from build123d import *

# Parameters (mm, degrees)
SKETCH1_R           = 20
SKETCH1_R_2         = 10
BOSS_EXTRUDE1_DEPTH = 10
SKETCH5_R           = 16.925
BOSS_EXTRUDE2_DEPTH = 20
BOSS_EXTRUDE3_DEPTH = 40
CIRPATTERN1_COUNT   = 4


with BuildPart() as part:
    # Sketch1 → Boss-Extrude1 (new, symmetric)
    with BuildSketch(Plane.XY):
        Circle(SKETCH1_R)
        Circle(SKETCH1_R_2, mode=Mode.SUBTRACT)
    extrude(amount=BOSS_EXTRUDE1_DEPTH, both=True)

    # Sketch5 → Boss-Extrude2 (add, symmetric)
    with BuildSketch(Plane.XY.offset(10)):
        Circle(SKETCH5_R)
    extrude(amount=BOSS_EXTRUDE2_DEPTH, both=True)

    # Sketch6 → Boss-Extrude3 (add)
    with BuildSketch(Plane(origin=(0, 0, 0), x_dir=(0, 0, -1), z_dir=(1, 0, 0))):
        Polygon((10, 0), (-10, 20), (-10, 17), (10, -3), align=None)
    boss_extrude3 = extrude(amount=BOSS_EXTRUDE3_DEPTH)

    # CirPattern1: Boss-Extrude3 ×4 about axis
    cirpattern1_axis = Axis((1.370302178, -0.068730139, 0), (0, 0, 1))
    for i in range(1, CIRPATTERN1_COUNT):
        add(boss_extrude3.rotate(cirpattern1_axis, i * 360 / CIRPATTERN1_COUNT))


solid = part.part
Geometry check sheet. Reference: the model listing, model coordinates, mm. A direction names the side the tool comes from. Round coordinates to 2 decimals unless told otherwise and drop trailing zeros. Order: outer loops, then holes, each group sorted by start corner. A loop starts at its lowest first (then second) coordinate and runs counter-clockwise, first axis right, second up. Notation, with made-up numbers: M -29.75,31.5 L -6.75,31.5 A24 cw -6.75,50.5 Z; hole C -10.75,-26 d10. An arc over 180 degrees is marked long. Write each question's results on one line, items separated by ' | '. Start each with the question number.
1. Set-up check for faces 4 (the face through (13, -11.3, 10)), 5 (the face through (0, 0, 30)): record each of +Z, -Z, +X, -X, +Y, -Y from which the full face is reachable in a straight line by a thin tool's end or side.
2. Material ranges on L1, parallel to Z at x = -10, y = 28.5; L2, parallel to Y at x = -1.5, z = 6.5; L3, parallel to Z at x = 11, y = -14, recorded low to high. Write a range as from..to.
3. Cross-section at D-D on y = -21.5. Record the boundary of the cut face in (x, z).
4. Cross-section at B-B on y = -12.5. Record the boundary of the cut face in (x, z), plus the area to 3 significant figures.
5. Cross-section at C-C on z = 21.5. Record the boundary of the cut face in (x, y) (3 decimals), plus the area to 3 significant figures.
6. Cross-section at A-A on x = -14.5. Record the boundary of the cut face in (y, z), plus the area to 3 significant figures.
7. Draft check along Z on faces 1 (the face through (6.88, 18.78, 0.14)), 2 (the face through (-8.6, 26.1, -0.1)), 3 (the face through (40, 9, 0)). Enter one of: pulls with the +Z half, pulls with the -Z half, needs draft (parallel to the pull), parting line crosses it, or undercut.
8. Go/stop test with flat-tipped pins: P1, Ø6, axis at y = 1.5, z = 10.5, coming from the -X side; P2, Ø6, axis at y = 6.5, z = 7.5, coming from the -X side; P3, Ø6, axis at x = 25, y = 6, coming from the +Z side. Record where each tip stops, or that it passes through.
Resolved:
1) face 4: +Z | face 5: +Z, +X, -X, +Y, -Y
2) L1: 1.3..4.3 | L2: -19.94..19.94 | L3: -10..10
3) outline: M -1.56,-10 L 1.44,-10 L 21.44,10 L 18.44,10 Z
4) outline: M -37.26,2.36 L -15.61,2.36 L -15.61,-10 L 15.61,-10 L 15.61,4.17 L 21.44,10 L 18.44,10 L 15.61,7.17 L 15.61,10 L 11.41,10 L 11.41,30 L -11.41,30 L -11.41,10 L -15.61,10 L -15.61,5.36 L -37.26,5.36 Z | area: 1,160 mm2
5) outline: C 0,0 d33.85 | area: 900 mm2
6) outline: M -20.14,10 L -13.77,3.64 L -13.77,-10 L 13.77,-10 L 13.77,5.8 L 38.56,5.8 L 38.56,8.8 L 13.77,8.8 L 13.77,10 L 8.73,10 L 8.73,30 L -8.73,30 L -8.73,10 L -13.77,10 L -13.77,6.64 L -17.14,10 Z | area: 989 mm2
7) face 1: undercut | face 2: pulls with the -Z half | face 3: needs draft
8) P1: x = -20 | P2: x = -19.69 | P3: z = 2
